from build123d import *

# Parameters (mm, degrees)
BOSS_EXTRUDE2_DEPTH = 37
BOSS_EXTRUDE4_DEPTH = 3
FILLET1_R           = 6.5
SKETCH5_R           = 2.1
CUT_EXTRUDE1_DEPTH  = 5
SKETCH6_W           = 50
SKETCH6_H           = 37
SKETCH6_W_2         = 46.2
SKETCH6_H_2         = 33.5
BOSS_EXTRUDE5_DEPTH = 5
SKETCH7_R           = 1.1
CUT_EXTRUDE2_DEPTH  = 1
CUT_EXTRUDE3_DEPTH  = 3
SKETCH9_R           = 5
CUT_EXTRUDE4_DEPTH  = 18.515687401
FILLET2_R           = 2


with BuildPart() as part:
    # Sketch2 → Boss-Extrude2 (new body)
    with BuildSketch(Plane(origin=(0, 0, 0), x_dir=(1, 0, 0), z_dir=(0, 1, 0))):
        with BuildLine():
            Line((32.692458993, 18.875), (34.857522502, 20.125))
            ThreePointArc((34.857522502, 20.125), (30.468551498, 26.300757966), (25, 31.544611267))
            Line((25, 31.544611267), (25, 40.390687301))
            Line((25, 40.390687301), (-25, 40.390687301))
            Line((-25, 40.390687301), (-25, 31.544611267))
            ThreePointArc((-25, 31.544611267), (-30.468551498, 26.300757966), (-34.857522502, 20.125))
            Line((-34.857522502, 20.125), (-32.692458993, 18.875))
            ThreePointArc((-32.692458993, 18.875), (0, 37.75), (32.692458993, 18.875))
        make_face()
    extrude(amount=BOSS_EXTRUDE2_DEPTH)

    # Sketch4 → Boss-Extrude4 (add)
    with BuildSketch(Plane(origin=(0, 37, 0), x_dir=(1, 0, 0), z_dir=(0, 1, 0))):
        with BuildLine():
            Line((-32.692458993, 18.875), (32.692458993, 18.875))
            Line((32.692458993, 18.875), (34.857522502, 20.125))
            ThreePointArc((34.857522502, 20.125), (0, 40.25), (-34.857522502, 20.125))
            Line((-34.857522502, 20.125), (-32.692458993, 18.875))
        make_face()
    extrude(amount=-BOSS_EXTRUDE4_DEPTH)

    # Fillet1
    fillet1_edges = [part.edges().sort_by_distance(p)[0] for p in [
        (0, 34, -37.75),
    ]]
    fillet(fillet1_edges, radius=FILLET1_R)

    # Sketch5 → Cut-Extrude1 (cut)
    with BuildSketch(Plane(origin=(0, 34, 0), x_dir=(-1, 0, 0), z_dir=(0, -1, 0))):
        with Locations((-6, 27)):
            Circle(SKETCH5_R)
        with Locations((6, 27)):
            Circle(SKETCH5_R)
    extrude(amount=-CUT_EXTRUDE1_DEPTH, mode=Mode.SUBTRACT)

    # Sketch6 → Boss-Extrude5 (add)
    with BuildSketch(Plane(origin=(0, 0, -40.390687301), x_dir=(-1, 0, 0), z_dir=(0, 0, -1))):
        with Locations((0, 18.5)):
            Rectangle(SKETCH6_W, SKETCH6_H)
        with Locations((0, 18.5)):
            Rectangle(SKETCH6_W_2, SKETCH6_H_2, mode=Mode.SUBTRACT)
    extrude(amount=BOSS_EXTRUDE5_DEPTH)

    # Sketch7 → Cut-Extrude2 (cut)
    with BuildSketch(Plane(origin=(0, 0, -40.390687301), x_dir=(-1, 0, 0), z_dir=(0, 0, -1))):
        with Locations((-18, 18.5)):
            Circle(SKETCH7_R)
        with Locations((18, 18.5)):
            Circle(SKETCH7_R)
    extrude(amount=-CUT_EXTRUDE2_DEPTH, mode=Mode.SUBTRACT)

    # Sketch8 → Cut-Extrude3 (cut)
    with BuildSketch(Plane(origin=(0, 0, -39.390687301), x_dir=(-1, 0, 0), z_dir=(0, 0, -1))):
        Polygon((-16, 17.345299462), (-16, 19.654700538), (-18, 20.809401077), (-20, 19.654700538), (-20, 17.345299462), (-18, 16.190598923), align=None)
        Polygon((20, 17.345299462), (20, 19.654700538), (18, 20.809401077), (16, 19.654700538), (16, 17.345299462), (18, 16.190598923), align=None)
    extrude(amount=-CUT_EXTRUDE3_DEPTH, mode=Mode.SUBTRACT)

    # Sketch9 → Cut-Extrude4 (cut, through all)
    with BuildSketch(Plane(origin=(0, 0, -36.390687301), x_dir=(-1, 0, 0), z_dir=(0, 0, -1))):
        with Locations((-18, 18.5)):
            Circle(SKETCH9_R)
        with Locations((18, 18.5)):
            Circle(SKETCH9_R)
    extrude(amount=-CUT_EXTRUDE4_DEPTH, mode=Mode.SUBTRACT)

    # Fillet2
    fillet2_edges = [part.edges().sort_by_distance(p)[0] for p in [
        (34.857522502, 18.5, -20.125),
        (-34.857522502, 18.5, -20.125),
        (-30.468551498, 37, -26.300757966),
        (-33.774990748, 37, -19.5),
        (33.774990748, 37, -19.5),
        (30.468551498, 37, -26.300757966),
    ]]
    fillet(fillet2_edges, radius=FILLET2_R)


solid = part.part
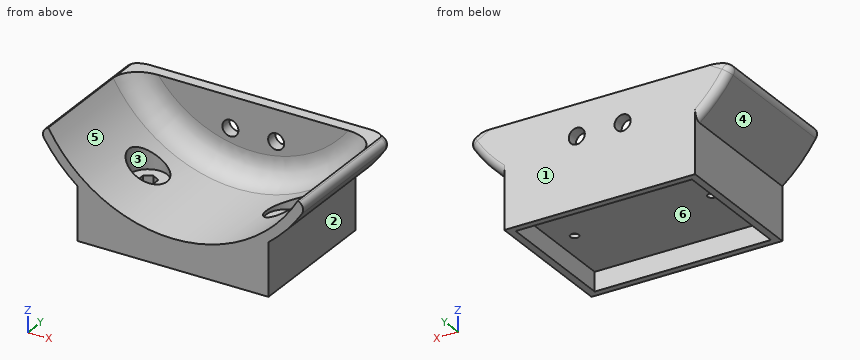
CAD build for the part. Positions are in the model's coordinates, mm. Face numbers are marked on the shaded views. A direction names the side the tool comes from. Coordinates: 2 decimals unless noted, no trailing zeros. Order: outer loops, then holes, each group sorted by start corner. A loop starts at its lowest first (then second) coordinate and runs counter-clockwise, first axis right, second up.
Item 1: 3-axis set-ups, long thin cutter, end or side, ignore diameter. For the marked faces 4, 5 and 6: which of +Z, -Z, +X, -X, +Y, -Y reach the whole face in a straight line?
Check sheet entries:
face 4: -Z, -X, +Y, -Y
face 5: +Z, -Y
face 6: -Z
Item 2: Drill centre lines: L1, parallel to Y at x = -18, z = -34.25; L2, parallel to X at y = 35.85, z = -27; L3, parallel to Y at x = 11, z = -43.75. Where is each one in solid material? Low to high.
Check sheet entries:
L1: y = 0 to 13.5, 23.5 to 37
L2: x = -29.59 to -8.1, -3.9 to 3.9, 8.1 to 29.59
L3: y = 0 to 1.75, 35.25 to 37
Item 3: Band-saw the part on A-A on y = 11. List the corners of the cut face in (x, z) (3 decimals), plus the area to 3 significant figures.
Check sheet entries:
outline: (-33.758, -21.92) arc R40.25 ccw to (-25, -31.545) - (-25, -45.391) - (-23.1, -45.391) - (-23.1, -40.391) - (23.1, -40.391) - (23.1, -45.391) - (25, -45.391) - (25, -31.545) arc R40.25 ccw to (33.758, -21.92) arc R2 ccw to (33.08, -19.099) - (32.692, -18.875) arc R37.75 cw to (-32.692, -18.875) - (-33.08, -19.099) arc R2 ccw to start
area: 367 mm2
Item 4: Pin check, flat tips, straight feed: pin 1 Ø1.5 at (x, y) = (-3.5, 32.5) entering from -Z; pin 2 Ø1.5 at (y, z) = (20.5, -27) entering from +X; pin 3 Ø3.5 at (x, z) = (-9, -25) entering from -Y; pin 4 Ø4 at (x, z) = (6, -27) entering from +Y. Stop position of each tip, or through.
Check sheet entries:
pin 1: stops at z = -40.39
pin 2: stops at x = 30.51
pin 3: stops at y = 34
pin 4: passes through
Item 5: Two-plate mould, pull along X, no slides. Class the marked faces 1, 2 and 3: +X half, -X half, draft (parallel to the pull), parting line (faces both ways), or undercut.
Check sheet entries:
face 1: draft
face 2: +X half
face 3: undercut
Item 6: Band-saw the part on B-B on y = 18.5. Give the number of separate pieces and of enclosed holes in the cut face, plus the area to 3 significant figures.
Check sheet entries:
separate pieces: 3
enclosed holes: 0
area: 271 mm2
Item 7: Band-saw the part on D-D on y = 29. List the corners of the cut face in (x, z) (3 decimals), plus the area to 3 significant figures.
Check sheet entries:
outline: (-33.758, -21.92) arc R40.25 ccw to (-25, -31.545) - (-25, -45.391) - (-23.1, -45.391) - (-23.1, -40.391) - (23.1, -40.391) - (23.1, -45.391) - (25, -45.391) - (25, -31.545) arc R40.25 ccw to (33.758, -21.92) arc R2 ccw to (33.08, -19.099) - (32.692, -18.875) - (32.49, -18.875) arc R37.575 cw to (-32.49, -18.875) - (-32.692, -18.875) - (-33.08, -19.099) arc R2 ccw to start
area: 380 mm2
